from build123d import *

# Parameters (mm, degrees)
SKETCH2_W            = 43.7
SKETCH2_H            = 47.2
SKETCH2_W_2          = 39.7
SKETCH2_H_2          = 42.879633868
SKETCH2_W_3          = 10
BOSS_EXTRUDE1_DEPTH  = 2
SKETCH3_W            = 47.7
SKETCH3_H            = 51.2
SKETCH3_W_2          = 43.7
SKETCH3_H_2          = 47.2
BOSS_EXTRUDE2_DEPTH  = 17
M6_CLEARANCE_HOLE1_D = 7
M6_CLEARANCE_HOLE2_D = 7
SKETCH9_W            = 5.969043329
SKETCH9_H            = 51.2
BOSS_EXTRUDE3_DEPTH  = 20
M5_CLEARANCE_HOLE1_D = 5.8
FILLET1_R            = 7.5
FILLET2_R            = 1
SKETCH15_W           = 14.80289281
SKETCH15_H           = 51.2
CUT_EXTRUDE1_DEPTH   = 41.301147626
SKETCH19_W           = 35.398634532
SKETCH19_H           = 47.4
CUT_EXTRUDE2_DEPTH   = 15


with BuildPart() as part:
    # Sketch2 → Boss-Extrude1 (new body)
    # profile 1 of 2: a face of its own
    with BuildSketch(Plane.XY):
        Rectangle(SKETCH2_W, SKETCH2_H)
        Rectangle(SKETCH2_W_2, SKETCH2_H_2, mode=Mode.SUBTRACT)
    # profile 2 of 2: a face of its own
    with BuildSketch(Plane.XY):
        with Locations((14.85, 0)):
            Rectangle(SKETCH2_W_3, SKETCH2_H_2)
    extrude(amount=BOSS_EXTRUDE1_DEPTH)

    # Sketch3 → Boss-Extrude2 (add)
    with BuildSketch(Plane.XY.offset(2)):
        Rectangle(SKETCH3_W, SKETCH3_H)
        Rectangle(SKETCH3_W_2, SKETCH3_H_2, mode=Mode.SUBTRACT)
    extrude(amount=-BOSS_EXTRUDE2_DEPTH)

    # M6 Clearance Hole1 (through all)
    with Locations(Plane(origin=(0, -25.6, 0), x_dir=(-1, 0, 0), z_dir=(0, -1, 0))):
        with Locations((0, 9)):
            Hole(M6_CLEARANCE_HOLE1_D / 2)

    # M6 Clearance Hole2 (through all)
    with Locations(Plane(origin=(23.85, 0, 0), x_dir=(0, 0, -1), z_dir=(1, 0, 0))):
        with Locations((9, 0)):
            Hole(M6_CLEARANCE_HOLE2_D / 2)

    # Sketch9 → Boss-Extrude3 (add)
    with BuildSketch(Plane.XY.offset(2)):
        with Locations((20.865478336, 0)):
            Rectangle(SKETCH9_W, SKETCH9_H)
    extrude(amount=BOSS_EXTRUDE3_DEPTH)

    # M5 Clearance Hole1 (through all)
    with Locations(Plane(origin=(23.85, 0, 0), x_dir=(0, 0, -1), z_dir=(1, 0, 0))):
        with Locations((-9.5, -15.6), (-9.5, 15.6), (-17, 0)):
            Hole(M5_CLEARANCE_HOLE1_D / 2)

    # Fillet1
    fillet1_edges = [part.edges().sort_by_distance(p)[0] for p in [
        (20.865478335, 25.6, 22),
        (20.865478335, -25.6, 22),
    ]]
    fillet(fillet1_edges, radius=FILLET1_R)

    # Fillet2
    fillet2_edges = [part.edges().sort_by_distance(p)[0] for p in [
        (0, 25.6, -15),
        (0, -25.6, -15),
    ]]
    fillet(fillet2_edges, radius=FILLET2_R)

    # Sketch15 → Cut-Extrude1 (cut, through all)
    with BuildSketch(Plane.XY.offset(2)):
        with Locations((-16.448553595, 0)):
            Rectangle(SKETCH15_W, SKETCH15_H)
    extrude(amount=-CUT_EXTRUDE1_DEPTH, mode=Mode.SUBTRACT)

    # Sketch19 → Cut-Extrude2 (cut)
    with BuildSketch(Plane(origin=(0, 0, -15), x_dir=(-1, 0, 0), z_dir=(0, 0, -1))):
        with Locations((-4.150682734, 0)):
            Rectangle(SKETCH19_W, SKETCH19_H)
    extrude(amount=-CUT_EXTRUDE2_DEPTH, mode=Mode.SUBTRACT)


solid = part.part
Source: CAD feature listing. Evaluate the final solid. Frame: model axes, mm. A direction names the side the tool comes from. Round coordinates to 2 decimals unless told otherwise and drop trailing zeros. Loops run counter-clockwise (first coordinate to the right, second up) from the corner with the lowest first, then second, coordinate; pieces in that order, holes last. Notation, with made-up numbers: (74.5, 37.5) - (109.5, 37.5) arc R21 cw to (109.5, 72.5) - close; hole circle Ø6 at (3, -26). An arc over 180 degrees is marked (long way). Write item = value, one per line. Start each with the question number.
Item 1: Section query C-C on x = 9. Output: boundary loops of the cut face in (y, z), plus the area to 3 significant figures.
Item 2: Section query A-A on z = 9.5. Output: boundary loops of the cut face in (x, y).
Item 3: Mould query, pull axis Z, two halves, no side actions, for faces 4 (the face through (10, 0, 2)), 5 (the face through (-0.759, 24.663, -5.583)), 6 (the face through (7, 23.7, -8)). Classes: released by +Z, released by -Z, zero draft, split by the parting line, or undercut.
Item 4: First-contact query: pin 1 Ø10 at (y, z) = (5.5, 13.5) entering from -X; pin 2 Ø7.5 at (y, z) = (-3.5, -9.5) entering from -X; pin 3 Ø3.5 at (y, z) = (15.6, 9.5) entering from -X; pin 4 Ø4 at (x, y) = (15.5, -11.5) entering from +Z. Flat tips, straight axial feed; report the tip coordinate or a pass-through.
Item 5: Section query B-B on y = 13.5. Output: boundary loops of the cut face in (x, z), plus the area to 3 significant figures.
Item 6: Material intervals for line 1 (Y direction, x = 23, z = -9); line 2 (Y direction, x = 19.8, z = 9.5); line 3 (Y direction, x = 5.5, z = -9), sorted ascending.
Item 7: Reachability of faces 1 (the face through (21.85, 0, -4)), 2 (the face through (11, -25.6, -3)), 3 (the face through (9.85, 0, 1)) from +Z, -Z, +X, -X, +Y, -Y: full face, straight path, thin tool, end or side. Return the list, or none.
Item 8: Section query D-D on y = 0. Output: boundary loops of the cut face in (x, z).
Results list:
q1.outline = (-25.6, -14) arc R1 ccw to (-24.6, -15) - (-23.7, -15) - (-23.7, 0) - (-21.44, 0) - (-21.44, 2) - (-25.6, 2) - close; (21.44, 0) - (23.7, 0) - (23.7, -15) - (24.6, -15) arc R1 ccw to (25.6, -14) - (25.6, 2) - (21.44, 2) - close
q1.area = 73.2 mm²
q2.outline = (17.88, -25.6) - (23.85, -25.6) - (23.85, -18.5) - (17.88, -18.5) - close; (17.88, -12.7) - (23.85, -12.7) - (23.85, 12.7) - (17.88, 12.7) - close; (17.88, 18.5) - (23.85, 18.5) - (23.85, 25.6) - (17.88, 25.6) - close
q3.face_4 = released by +Z
q3.face_5 = undercut
q3.face_6 = zero draft
q4.pin_1 = 17.88
q4.pin_2 = 21.85
q4.pin_3 = through
q4.pin_4 = 2
q5.outline = (9.85, 0) - (21.85, 0) - (21.85, -15) - (23.85, -15) - (23.85, 7.5) - (17.88, 7.5) - (17.88, 2) - (9.85, 2) - close; (17.88, 11.5) - (23.85, 11.5) - (23.85, 22) - (17.88, 22) - close
q5.area = 154 mm²
q6.line_1 = -25.6 to -3.5, 3.5 to 25.6
q6.line_2 = -25.6 to -18.5, -12.7 to 12.7, 18.5 to 25.6
q6.line_3 = -25.6 to -23.7, 23.7 to 25.6
q7.face_1 = -Z, -X
q7.face_2 = +Z, -Z, +X, -X, -Y
q7.face_3 = +Z, -Z, -X
q8.outline = (9.85, 0) - (21.85, 0) - (21.85, -5.5) - (23.85, -5.5) - (23.85, 14.1) - (17.88, 14.1) - (17.88, 2) - (9.85, 2) - close; (17.88, 19.9) - (23.85, 19.9) - (23.85, 22) - (17.88, 22) - close; (21.85, -15) - (23.85, -15) - (23.85, -12.5) - (21.85, -12.5) - close
